from build123d import *

# Parameters (mm, degrees)
SKETCH1_R           = 7.9
SKETCH1_R_2         = 9
SKETCH1_R_3         = 2.5
SKETCH1_R_4         = 4
BOSS_EXTRUDE1_DEPTH = 4


with BuildPart() as part:
    # Sketch1 → Boss-Extrude1 (new body)
    with BuildSketch(Plane.XY):
        with BuildLine():
            Line((0, 0), (120, 0))
            Line((120, 0), (120, 90))
            ThreePointArc((120, 90), (117.071067812, 97.071067812), (110, 100))
            Line((110, 100), (10, 100))
            ThreePointArc((10, 100), (2.928932188, 97.071067812), (0, 90))
            Line((0, 90), (0, 0))
        make_face()
        with Locations((100, 85)):
            Circle(SKETCH1_R, mode=Mode.SUBTRACT)
        with Locations((20, 85)):
            Circle(SKETCH1_R, mode=Mode.SUBTRACT)
        with Locations((50.040016013, 50)):
            Circle(SKETCH1_R_2, mode=Mode.SUBTRACT)
        with Locations((58.359688144, 38.124266101)):
            Circle(SKETCH1_R_3, mode=Mode.SUBTRACT)
        with Locations((41.720343882, 61.875733899)):
            Circle(SKETCH1_R_3, mode=Mode.SUBTRACT)
        with Locations((100, 20)):
            Circle(SKETCH1_R_4, mode=Mode.SUBTRACT)
        with Locations((20, 20)):
            Circle(SKETCH1_R_4, mode=Mode.SUBTRACT)
        with BuildLine():
            ThreePointArc((38.959835733, 20), (60, 11.284878606), (81.040164267, 20))
            ThreePointArc((81.040164267, 20), (84.575698173, 20), (84.575698173, 16.464466094))
            ThreePointArc((84.575698173, 16.464466094), (60, 6.284878606), (35.424301827, 16.464466094))
            ThreePointArc((35.424301827, 16.464466094), (35.424301827, 20), (38.959835733, 20))
        make_face(mode=Mode.SUBTRACT)
    extrude(amount=BOSS_EXTRUDE1_DEPTH)


solid = part.part
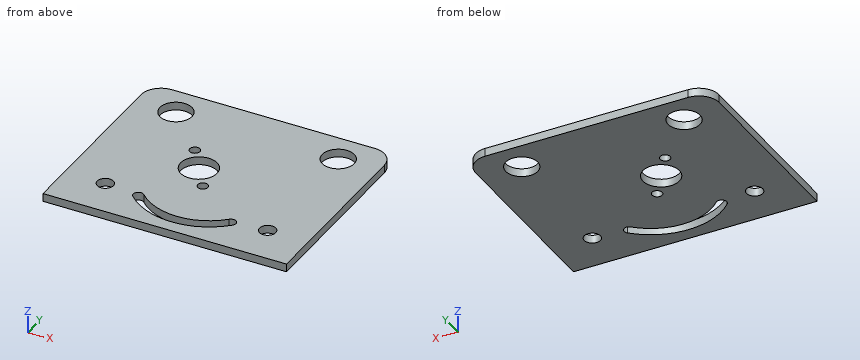
Verification items for the finished model (mm, model axes). Coordinates: 2 decimals unless noted, no trailing zeros. Order: outer loops, then holes, each group sorted by start corner. A loop starts at its lowest first (then second) coordinate and runs counter-clockwise, first axis right, second up. Notation, with made-up numbers: M 35.25,-11 L 80.25,-11 A14 ccw 80.25,7 Z; hole C 73.25,18 d11. An arc over 180 degrees is marked long. Write each question's results on one line, items separated by ' | '.
1) Section check D-D on z = 1.8. Give the number of separate pieces and of enclosed holes in the cut face, plus the area to 3 significant figures.
Solved:
separate pieces: 1 | enclosed holes: 8 | area: 10,900 mm²
2) Scan lines: line 1 along Y through (x, z) = (20, 2); line 2 along X through (y, z) = (89, 2.9); line 3 along Y through (x, z) = (44, 0.4). Record each from-to range of solid material in increasing order. Write a range as [from, to].
Solved:
line 1: y = [0, 16], [24, 77.1], [92.9, 100] | line 2: x = [0, 13.19], [26.81, 93.19], [106.81, 120] | line 3: y = [0, 10.19], [15.95, 43.33], [56.67, 60.85], [62.9, 100]
3) Section check C-C on y = 85. Record the cut outline in (x, z).
Solved:
outline: M 0,0 L 12.1,0 L 12.1,4 L 0,4 Z; M 27.9,0 L 92.1,0 L 92.1,4 L 27.9,4 Z; M 107.9,0 L 120,0 L 120,4 L 107.9,4 Z
4) Section check B-B on x = 100. Record the cut outline in (y, z), plus the area to 3 significant figures.
Solved:
outline: M 0,0 L 16,0 L 16,4 L 0,4 Z; M 24,0 L 77.1,0 L 77.1,4 L 24,4 Z; M 92.9,0 L 100,0 L 100,4 L 92.9,4 Z | area: 305 mm²
5) Gauge pin test, flat end, axial feed: pin 1 Ø4.5 at (x, y) = (58.36, 38.12) entering from -Z. Record the tip position at first contact, or that the pin passes through.
Solved:
pin 1: passes through
6) Section check A-A on y = 50. Record the cut outline in (x, z), plus the area to 3 significant figures.
Solved:
outline: M 0,0 L 41.04,0 L 41.04,4 L 0,4 Z; M 59.04,0 L 120,0 L 120,4 L 59.04,4 Z | area: 408 mm²
